Autodesk Inventor part; units mm, degrees
ref_plane "Work Plane1" through (0, 0, 0) normal (1, 0, 0) x (0, 1, 0)
ref_plane "Work Plane2" through (0, 0, 0) normal (0, 1, 0) x (1, 0, 0)
ref_plane "XY Plane" through (0, 0, 0) normal (0, 0, 1) x (1, 0, 0)
sketch "Sketch1" plane through (0, 0, 0) normal (0, 0, 1) x (1, 0, 0)
  line L0 (6.5405, -6.5405) -> (-6.5405, -6.5405)
  line L1 (-6.5405, -6.5405) -> (-6.5405, 6.5405)
  line L2 (-6.5405, 6.5405) -> (6.5405, 6.5405)
  line L3 (6.5405, 6.5405) -> (6.5405, -6.5405)
  line L4 (6.5405, -6.5405) -> (-6.5405, 6.5405) construction
  line L5 (-6.5405, -6.5405) -> (6.5405, 6.5405) construction
  circle A0 centre (0, 0) radius 2.413
  dimension "d0" = 13.081
  dimension "d1" = 4.826
extrude "Extrusion1" add sketch "Sketch1" along normal blind 152.4
sketch "Sketch2" plane through (0, 0, 152.4) normal (0, 0, 1) x (1, 0, 0)
  circle A0 centre (0, 0) radius 2.413
  line L0 (6.5405, -6.5405) -> (6.5405, 6.5405)
  line L1 (19.05, 19.05) -> (19.05, 4.445)
  line L2 (19.05, 4.445) -> (15.24, 4.445)
  line L3 (11.9561, 10.16) -> (6.5405, 4.7444)
  line L4 (15.24, 4.445) -> (15.24, 6.985)
  line L5 (15.24, 6.985) -> (16.002, 6.985)
  line L6 (16.002, 6.985) -> (16.002, 10.16)
  line L7 (16.002, 10.16) -> (11.9561, 10.16)
  line L8 (19.05, 19.05) -> (6.5405, 6.5405) construction
  line L9 (19.05, 19.05) -> (4.445, 19.05)
  line L10 (4.445, 19.05) -> (4.445, 15.24)
  line L11 (10.16, 11.9561) -> (4.7444, 6.5405)
  line L12 (4.445, 15.24) -> (6.985, 15.24)
  line L13 (6.985, 15.24) -> (6.985, 16.002)
  line L14 (6.985, 16.002) -> (10.16, 16.002)
  line L15 (10.16, 16.002) -> (10.16, 11.9561)
  line L16 (4.7444, 6.5405) -> (6.5405, 6.5405)
  line L17 (6.5405, 6.5405) -> (6.5405, 4.7444)
  dimension "d5" = 45
  dimension "d6" = 14.605
  dimension "d7" = 3.81
  dimension "d8" = 3.048
  dimension "d10" = 19.05
  dimension "d13" = 8.89
  dimension "d14" = 1.27
  dimension "d15" = 3.175
extrude "Extrusion2" add sketch "Sketch2" against normal up to surface (152.4 mm away) contours L0 L16 L11 L15 L14 L13 L12 L10 L9 L1 L2 L4 L5 L6 L7 L3
pattern_circular "Circular Pattern1" count 4 over 360 about axis through (0, 0, 0) along (0, 0, 1) of "Extrusion2"
ref_plane "Work Plane1" through (0, 0, 0) normal (1, 0, 0) x (0, 1, 0)
ref_plane "Work Plane2" through (0, 0, 0) normal (0, 1, 0) x (1, 0, 0)
equation "\"d10\" = d9"
properties part number "1_5 80-20 x 6in" material "Gold"
The listing builds one solid part. Answer for the finished solid, in the listing's coordinates (mm). A direction names the side the tool comes from. Coordinates: 2 decimals unless noted, no trailing zeros. Write each loop counter-clockwise with the first axis right and the second up, starting at its lowest first coordinate (ties: lowest second). Pieces come first, ordered by that corner, then holes. Notation, with made-up numbers: (80, 20) - (89, 20) arc R21 cw to (89, 57) - close; hole circle Ø3 at (85, 88.25). An arc over 180 degrees is marked (long way). Return JSON: item names as keys, results as strings. Group by question number.
Q1. Which of the six approach directions +Z, -Z, +X, -X, +Y, -Y give full straight-line access (tool end or side, diameter ignored) to faces 1 (the flat face through (16.002, -9, 77)), 2 (the flat face through (-17, -4.445, 77)), 3 (the flat face through (19.05, -12, 77))?
Q2. Find the intervals of material crossed by line 1 along Y through (x, z) = (0, 107); line 2 along X through (y, z) = (5, 130); line 3 along Y through (x, z) = (-9, 130.5), in increasing order. Write a range as [from, to].
Q3. The part is cut by section A-A on x = 0. Write down the section's boundary in (y, z).
Q4. Flat-ended cylindrical pins translate along their axes: pin 1 Ø3 at (x, y) = (-3.5, -8.5) entering from -Z; pin 2 Ø4.5 at (x, z) = (-1, 104.5) entering from -Y; pin 3 Ø7.5 at (y, z) = (0.5, 89.5) entering from -X. Find the tip coordinate at first contact, or state that the pin passes through.
Evaluation:
{
 "1": {"face 1": "+Z, -Z", "face 2": "+Z, -Z, -X", "face 3": "+Z, -Z, +X, +Y, -Y"},
 "2": {"line 1": "y = [-6.54, -2.41], [2.41, 6.54]", "line 2": "x = [-19.05, -15.24], [-6.8, 6.8], [15.24, 19.05]", "line 3": "y = [-19.05, -16], [-10.8, -7.2], [7.2, 10.8], [16, 19.05]"},
 "3": {"outline": "(-6.54, 0) - (-2.41, 0) - (-2.41, 152.4) - (-6.54, 152.4) - close; (2.41, 0) - (6.54, 0) - (6.54, 152.4) - (2.41, 152.4) - close"},
 "4": {"pin 1": "passes through", "pin 2": "stops at y = -6.54", "pin 3": "stops at x = -6.54"}
}
